Read the model definition and answer for the solid it produces. Units are mm, in the model's axes. Round coordinates to 2 decimals unless told otherwise and drop trailing zeros. Loops run counter-clockwise (first coordinate to the right, second up) from the corner with the lowest first, then second, coordinate; pieces in that order, holes last. Notation, with made-up numbers: (53.25, 76.25) -> (109.25, 76.25) arc R13 ccw to (109.25, 93.25) -> close; hole circle Ø10 at (-23.5, 88.5). An arc over 180 degrees is marked (long way). Put each result on its own line as item: value.
from build123d import *

# Parameters (mm, degrees)
SKETCH1_W           = 43.18
SKETCH1_H           = 57.15
BOSS_EXTRUDE1_DEPTH = 6.35
SKETCH2_R           = 1.651
CUT_EXTRUDE1_DEPTH  = 53.459609614
CUT_EXTRUDE2_DEPTH  = 53.459609614


with BuildPart() as part:
    # Sketch1 → Boss-Extrude1 (new body)
    with BuildSketch(Plane(origin=(0, 0, 0), x_dir=(1, 0, 0), z_dir=(0, 1, 0))):
        Polygon((-31.75, -20.955), (-21.59, -15.718655855), (-21.59, -8.411344145), (-31.75, -3.175), align=None)
        Rectangle(SKETCH1_W, SKETCH1_H)
        Polygon((-31.75, 3.175), (-21.59, 8.411344145), (-21.59, 15.718655855), (-31.75, 20.955), align=None)
        with BuildLine():
            Line((-4.218626538, -28.575), (-21.59, -28.575))
            Line((-21.59, -28.575), (-21.59, -41.275))
            add(Edge.make_bspline(
                [(-21.59, -41.275), (-17.723032693, -28.747286936), (-4.218626538, -28.575)],
                knots=[0, 0, 0, 0.972868199, 0.972868199, 0.972868199], degree=2))
        make_face()
        with BuildLine():
            Line((-21.59, 41.275), (-21.59, 28.575))
            Line((-21.59, 28.575), (-4.218626538, 28.575))
            add(Edge.make_bspline(
                [(-21.59, 41.275), (-17.723032693, 28.747286936), (-4.218626538, 28.575)],
                knots=[0, 0, 0, 0.972868199, 0.972868199, 0.972868199], degree=2))
        make_face()
    extrude(amount=BOSS_EXTRUDE1_DEPTH)

    # Sketch2 → Cut-Extrude1 (cut, through all)
    with BuildSketch(Plane(origin=(0, 6.35, 0), x_dir=(1, 0, 0), z_dir=(0, 1, 0))):
        with Locations(Location((4.2672, 24.003, 0), (0, 0, 270))):
            Circle(SKETCH2_R)
        with Locations(Location((4.2672, -24.003, 0), (0, 0, 270))):
            Circle(SKETCH2_R)
        with Locations(Location((10.6172, 24.003, 0), (0, 0, 270))):
            Circle(SKETCH2_R)
        with Locations(Location((10.6172, -24.003, 0), (0, 0, 270))):
            Circle(SKETCH2_R)
        with Locations(Location((16.9672, 24.003, 0), (0, 0, 270))):
            Circle(SKETCH2_R)
        with Locations(Location((16.9672, -24.003, 0), (0, 0, 270))):
            Circle(SKETCH2_R)
        with Locations(Location((-2.0828, 24.003, 0), (0, 0, 270))):
            Circle(SKETCH2_R)
        with Locations(Location((-2.0828, -24.003, 0), (0, 0, 270))):
            Circle(SKETCH2_R)
        with Locations(Location((-8.4328, 24.003, 0), (0, 0, 270))):
            Circle(SKETCH2_R)
        with Locations(Location((-8.4328, -24.003, 0), (0, 0, 270))):
            Circle(SKETCH2_R)
        with Locations(Location((-14.7828, 24.003, 0), (0, 0, 270))):
            Circle(SKETCH2_R)
        with Locations(Location((-14.7828, -24.003, 0), (0, 0, 270))):
            Circle(SKETCH2_R)
    extrude(amount=-CUT_EXTRUDE1_DEPTH, mode=Mode.SUBTRACT)

    # Sketch3 → Cut-Extrude2 (cut, through all)
    with BuildSketch(Plane(origin=(0, 6.35, 0), x_dir=(1, 0, 0), z_dir=(0, 1, 0))):
        Polygon((-17.387060633, 18.288), (-15.700620496, 21.209), (-19.05, 21.209), (-19.05, 18.288), align=None)
        Polygon((-4.335480447, 17.526), (-6.461861489, 21.209), (-13.940856876, 21.209), (-16.067237917, 17.526), (-13.13429855, 12.446), (-7.268419815, 12.446), align=None)
        Polygon((-17.387060633, 16.764), (-19.05, 16.764), (-19.05, 6.604), (-17.387060633, 6.604), (-14.454121265, 11.684), align=None)
        Polygon((-16.067237917, 5.842), (-13.13429855, 0.762), (-7.268419815, 0.762), (-4.335480447, 5.842), (-7.268419815, 10.922), (-13.13429855, 10.922), align=None)
        Polygon((-17.387060633, 5.08), (-19.05, 5.08), (-19.05, -5.08), (-17.387060633, -5.08), (-14.454121265, 0), align=None)
        Polygon((-16.067237917, -5.842), (-13.13429855, -10.922), (-7.268419815, -10.922), (-4.335480447, -5.842), (-7.268419815, -0.762), (-13.13429855, -0.762), align=None)
        Polygon((-19.05, -6.604), (-19.05, -16.764), (-17.387060633, -16.764), (-14.454121265, -11.684), (-17.387060633, -6.604), align=None)
        Polygon((-13.940856876, -21.209), (-6.461861489, -21.209), (-4.335480447, -17.526), (-7.268419815, -12.446), (-13.13429855, -12.446), (-16.067237917, -17.526), align=None)
        Polygon((-19.05, -21.209), (-15.700620496, -21.209), (-17.387060633, -18.288), (-19.05, -18.288), align=None)
        Polygon((-4.619379504, -21.209), (4.619379504, -21.209), (2.932939367, -18.288), (-2.932939367, -18.288), align=None)
        Polygon((-2.932939367, -16.764), (2.932939367, -16.764), (5.865878735, -11.684), (2.932939367, -6.604), (-2.932939367, -6.604), (-5.865878735, -11.684), align=None)
        Polygon((-2.932939367, -5.08), (2.932939367, -5.08), (5.865878735, 0), (2.932939367, 5.08), (-2.932939367, 5.08), (-5.865878735, 0), align=None)
        Polygon((-2.932939367, 6.604), (2.932939367, 6.604), (5.865878735, 11.684), (2.932939367, 16.764), (-2.932939367, 16.764), (-5.865878735, 11.684), align=None)
        Polygon((2.932939367, 18.288), (4.619379504, 21.209), (-4.619379504, 21.209), (-2.932939367, 18.288), align=None)
        Polygon((15.984519553, 17.526), (13.858138511, 21.209), (6.379143124, 21.209), (4.252762083, 17.526), (7.18570145, 12.446), (13.051580185, 12.446), align=None)
        Polygon((17.387060633, 18.288), (19.05, 18.288), (19.05, 21.209), (15.700620496, 21.209), align=None)
        Polygon((17.387060633, 6.604), (19.05, 6.604), (19.05, 16.764), (17.387060633, 16.764), (14.454121265, 11.684), align=None)
        Polygon((4.252762083, 5.842), (7.18570145, 0.762), (13.051580185, 0.762), (15.984519553, 5.842), (13.051580185, 10.922), (7.18570145, 10.922), align=None)
        Polygon((19.05, -5.08), (19.05, 5.08), (17.387060633, 5.08), (14.454121265, 0), (17.387060633, -5.08), align=None)
        Polygon((4.252762083, -5.842), (7.18570145, -10.922), (13.051580185, -10.922), (15.984519553, -5.842), (13.051580185, -0.762), (7.18570145, -0.762), align=None)
        Polygon((19.05, -16.764), (19.05, -6.604), (17.387060633, -6.604), (14.454121265, -11.684), (17.387060633, -16.764), align=None)
        Polygon((6.379143124, -21.209), (13.858138511, -21.209), (15.984519553, -17.526), (13.051580185, -12.446), (7.18570145, -12.446), (4.252762083, -17.526), align=None)
        Polygon((19.05, -21.209), (19.05, -18.288), (17.387060633, -18.288), (15.700620496, -21.209), align=None)
    extrude(amount=-CUT_EXTRUDE2_DEPTH, mode=Mode.SUBTRACT)


solid = part.part
Item 1: The part is cut by section C-C (y = 5.25). State how many separate pieces and enclosed holes the cut face has, then the cut area to 3 significant figures.
Derived:
separate pieces: 1
enclosed holes: 35
area: 1,520 mm^2
Item 2: Flat-ended cylindrical pins translate along their axes: pin 1 Ø1.8 at (x, y) = (18, 1.5) entering from +Z (3 decimals); pin 2 Ø3 at (x, y) = (10.5, 4.5) entering from -Z (3 decimals); pin 3 Ø0.5 at (x, y) = (-18.5, 4.5) entering from +Z; pin 4 Ø5 at (x, z) = (-23, 10.5) entering from -Y. Find the tip coordinate at first contact, or state that the pin passes through.
Derived:
pin 1: stops at z = 28.575
pin 2: stops at z = -28.575
pin 3: stops at z = 35.34
pin 4: stops at y = 0
Item 3: The part is cut by section A-A (x = -26.5). Determine the outline of the cut face in (y, z), then the cut area to 3 significant figures.
Derived:
outline: (0, -18.25) -> (6.35, -18.25) -> (6.35, -5.88) -> (0, -5.88) -> close; (0, 5.88) -> (6.35, 5.88) -> (6.35, 18.25) -> (0, 18.25) -> close
area: 157 mm^2
Item 4: The part is cut by section B-B (z = -27). Determine the outline of the cut face in (x, y), then the cut area to 3 significant figures.
Derived:
outline: (-21.59, 0) -> (21.59, 0) -> (21.59, 6.35) -> (-21.59, 6.35) -> close
area: 274 mm^2
Item 5: Find the intervals of material crossed by line 1 along Z through (x, y) = (0.5, 0.5) (3 decimals); line 2 along X through (y, z) = (0.75, 9); line 3 along X through (y, z) = (5, -15.5), in increasing order.
Derived:
line 1: z = -28.575 to -21.209, -18.288 to -16.764, -6.604 to -5.08, 5.08 to 6.604, 16.764 to 18.288, 21.209 to 28.575
line 2: x = -31.75 to -19.05, -16 to -14.24, -6.16 to -4.32, 4.32 to 6.08, 14.16 to 16, 19.05 to 21.59
line 3: x = -31.75 to -19.05, -16.66 to -14.9, -5.51 to -3.66, 3.66 to 5.42, 14.81 to 16.66, 19.05 to 21.59
